For this review, take the finished solid that the model builds, in its own axes (mm). Face numbers are marked on the shaded views. A direction names the side the tool comes from. Coordinates: 2 decimals unless noted, no trailing zeros. Write each loop counter-clockwise with the first axis right and the second up, starting at its lowest first coordinate (ties: lowest second). Pieces come first, ordered by that corner, then holes.
1) Mouldability with a two-part tool opening along Z and no side actions: class the marked faces 1, 2 and 3 as pulls with the +Z half, pulls with the -Z half, needs draft (parallel to the pull), parting line crosses it, or undercut.
2) For the marked faces 4 and 5, list the 3-axis set-ups (+Z, -Z, +X, -X, +Y, -Y) from which the entire face can be reached by the end or side of a thin tool; tool diameter is ignored.
3) We need section A-A on z = 14.35. Write out the cut boundary in (x, y), then the cut area to 3 significant figures.
4) Insertion check: P1, Ø1, axis at x = -11, z = 1, coming from the +Y side; P2, Ø3, axis at x = -13, y = 5.5, coming from the +Z side; P3, Ø5.5, axis at x = 0, y = -5.1, coming from the -Z side. Each pin has a flat end and moves straight along its axis. Give the tip position at first contact, or say it passes through.
5) To check wall thickness, follow line 1 along Y through (x, z) = (0, 32.55); line 2 along Y through (x, z) = (5, -3.4); line 3 along X through (y, z) = (-7.75, 24). State the ranges of each line that lie inside material, in increasing order.
6) We need section B-B on x = 0. Write out the cut boundary in (y, z).
7) We need section C-C on y = 13.25. Write out the cut boundary in (x, z) (3 decimals), then the cut area to 3 significant figures.
8) We need section D-D on x = 7. Write out the cut boundary in (y, z), then the cut area to 3 significant figures.
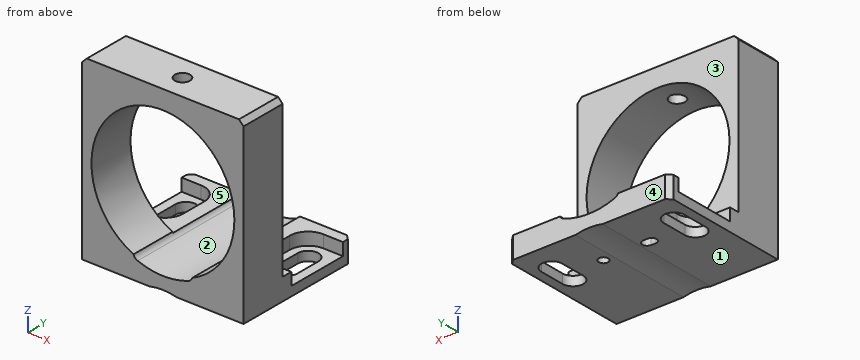
Autodesk Inventor part; units mm, degrees
ref_plane "YZ Plane" through (0, 0, 0) normal (1, 0, 0) x (0, 1, 0)
ref_plane "XZ Plane" through (0, 0, 0) normal (0, 1, 0) x (-1, 0, 0)
ref_plane "XY Plane" through (0, 0, 0) normal (0, 0, 1) x (1, 0, 0)
sketch "Sketch4" plane through (0, 0, 0) normal (0, 0, 1) x (1, 0, 0)
  line L0 (-17.54, 18) -> (17.54, 18)
  line L1 (17.54, 18) -> (17.54, -10.2)
  line L2 (17.54, -10.2) -> (-17.54, -10.2)
  line L3 (-17.54, -10.2) -> (-17.54, 18)
  point P0 (0, 0)
  dimension "d24" = 28.2
  dimension "WIDTH" = 35.08
  dimension "d26" = 17.54
  dimension "d28" = 10.2
extrude "Extrusion3" add sketch "Sketch4" against normal blind 4.7
sketch "Sketch5" plane through (0, 0, 0) normal (0, 0, 1) x (1, 0, 0)
  line L0 (-17.54, -10.2) -> (17.54, -10.2)
  line L1 (17.54, -10.2) -> (17.54, 0)
  line L2 (17.54, 0) -> (-17.54, 0)
  line L3 (-17.54, 0) -> (-17.54, -10.2)
  line L4 (-17.54, 18) -> (-17.54, -10.2)
  line L5 (-17.54, -10.2) -> (17.54, -10.2)
  line L6 (17.54, -10.2) -> (17.54, 18)
  point P0 (0, 0)
  dimension "d31" = 0
  dimension "d32" = 0
  dimension "d33" = 0
  dimension "d34" = 0
extrude "Extrusion4" add sketch "Sketch5" along normal blind 33.93
sketch "Sketch7" plane through (-17.54, -10.2, -4.7) normal (0, -1, 0) x (1, 0, 0)
  circle A0 centre (17.54, 19.05) radius 15.29
  line L0 (35.08, 0) -> (35.08, 38.63)
  line L1 (0, 38.63) -> (35.08, 38.63)
  line L2 (35.08, 0) -> (0, 0)
  line L3 (0, 38.63) -> (0, 0)
  circle A1 centre (17.54, 19.05) radius 15.79
  circle A2 centre (12.6611, 5.6453) radius 1.525
  circle A3 centre (22.4189, 5.6453) radius 1.525
  line L4 (17.54, 19.05) -> (17.54, 6.8001)
  line L5 (12.6611, 5.6453) -> (17.54, 19.05)
  line L6 (22.4189, 5.6453) -> (17.54, 19.05)
  point P0 (22.9405, 4.2123)
  point P1 (21.6565, 4.3246)
  point P2 (13.4235, 4.3246)
  point P3 (12.1395, 4.2123)
  point P4 (23.8519, 5.1236)
  point P5 (11.2281, 5.1236)
  dimension "PILOT_HOLE" = 30.58
  dimension "d201" = 19.05
  dimension "d225" = 17.54
  dimension "d226" = 31.58
  dimension "d227" = 20
  dimension "d228" = 20
  dimension "d229" = 3.05
  dimension "d230" = 3.05
  dimension "d231" = 14.265
  dimension "d232" = 14.265
sketch "Sketch9" plane through (0, 0, -4.7) normal (0, 0, -1) x (-1, 0, 0)
  line L0 (17.54, 18) -> (-17.54, 18)
  line L1 (17.54, 0) -> (-17.54, 0)
  line L2 (0, 5.488) -> (0, 10.988) construction
  line L3 (2.25, 5.488) -> (2.25, 10.988)
  line L4 (-2.25, 10.988) -> (-2.25, 5.488)
  arc A0 (-2.25, 5.488) -> (2.25, 5.488) centre (0, 5.488) ccw
  arc A1 (2.25, 10.988) -> (-2.25, 10.988) centre (0, 10.988) ccw
  line L5 (5.498, 8.238) -> (4.502, 8.238) construction
  line L6 (5.498, 9.288) -> (4.502, 9.288)
  line L7 (4.502, 7.188) -> (5.498, 7.188)
  arc A2 (5.498, 7.188) -> (5.498, 9.288) centre (5.498, 8.238) ccw
  arc A3 (4.502, 9.288) -> (4.502, 7.188) centre (4.502, 8.238) ccw
  point P0 (0, 0)
  point P1 (-5, 8.238)
  point P2 (0, 8.238)
  point P3 (5, 8.238)
  dimension "d183" = 18
  dimension "d185" = 2.25
  dimension "d186" = 5.5
  dimension "d187" = 0
  dimension "d188" = 8.238
  dimension "d189" = 1.05
  dimension "d190" = 0.996
  dimension "d191" = 0
  dimension "d192" = 5
  dimension "d203" = 0
  dimension "d204" = 5
extrude "Extrusion6" cut sketch "Sketch9" against normal blind 2.1 contours A2 L7 A3 L6
extrude "Extrusion7" cut sketch "Sketch7" against normal up to surface (10.2 mm away) contours A0 A3 L6 L5 A2 | A2 A0 | A0 A2 | A3 A0 | A0 A3 | A2 L5 L6 A3 A0 | A0 A3 A1 A2 picked at (17.54, 3.6354)
hole "Hole3" at (5, 8.238, -4.7) direction (0, 0, 1) diameter 2.1 depth 2.1
chamfer "Chamfer10" distance 1 angle 45 4 edges at (17.54, -5.1, 33.93) (-17.54, -5.1, 33.93) (17.54, 18, -2.35) (-17.54, 18, -2.35)
sketch "Sketch13" plane through (-16.54, 18, 0) normal (0, 1, 0) x (1, 0, 0)
  circle A0 centre (16.54, 17.05) radius 12.7
  line L0 (0, 4.7) -> (33.08, 4.7)
  point P0 (16.54, 0)
  dimension "d196" = 0
  dimension "d197" = 25.4
  dimension "d224" = 12.35
extrude "Extrusion11" cut sketch "Sketch13" against normal up to surface (28.2 mm away)
sketch "Sketch14" plane through (0, 0, 33.93) normal (0, 0, 1) x (1, 0, 0)
  line L0 (-17.54, -10.2) -> (17.54, -10.2)
  point P0 (0, 0)
  point P1 (0, -5.1)
  point P2 (-16.54, -10.2)
  point P3 (16.54, -10.2)
  dimension "d212" = 0
  dimension "d213" = 5.1
  dimension "d214" = 10.2
hole "Hole4" at (0, -5.1, 33.93) direction (0, 0, -1) diameter 3.302 end up to surface
sketch "Sketch20" plane through (0, 0, -4.7) normal (0, 0, -1) x (-1, 0, 0)
  line L0 (-17.54, 18) -> (17.54, 18)
  line L1 (-17.54, 0) -> (-17.54, 18)
  line L2 (-13.29, 6.25) -> (-13.29, 11.75) construction
  line L3 (-11.04, 6.25) -> (-11.04, 11.75)
  line L4 (-15.54, 11.75) -> (-15.54, 6.25)
  arc A0 (-15.54, 6.25) -> (-11.04, 6.25) centre (-13.29, 6.25) ccw
  arc A1 (-11.04, 11.75) -> (-15.54, 11.75) centre (-13.29, 11.75) ccw
  line L5 (5.2784, 0) -> (5.2784, 18)
  line L6 (17.54, 18) -> (-17.54, 18)
  line L7 (17.54, -10.2) -> (17.54, 18)
  line L8 (13.29, 6.25) -> (13.29, 11.75) construction
  line L9 (15.54, 6.25) -> (15.54, 11.75)
  line L10 (11.04, 11.75) -> (11.04, 6.25)
  arc A2 (11.04, 6.25) -> (15.54, 6.25) centre (13.29, 6.25) ccw
  arc A3 (15.54, 11.75) -> (11.04, 11.75) centre (13.29, 11.75) ccw
  circle A4 centre (-5, 8.238) radius 1.05
  point P0 (0, 0)
  point P1 (-13.29, 9)
  point P2 (-5.2784, 18)
  point P3 (17.54, 0)
  point P4 (13.29, 9)
  point P5 (16.54, 18)
  dimension "d251" = 18
  dimension "d252" = 9
  dimension "d253" = 12.2616
  dimension "d254" = 4.25
  dimension "d255" = 4.5
  dimension "d256" = 5.5
  dimension "d257" = 18
  dimension "d258" = 12.2616
  dimension "d259" = 9
  dimension "d261" = 4.5
  dimension "d262" = 5.5
  dimension "d293" = 4.25
extrude "Extrusion15" cut sketch "Sketch20" against normal through all contours A0 L4 A1 L3 | A2 L10 A3 L9
sketch "Sketch21" plane through (0, 0, 0) normal (0, 0, 1) x (1, 0, 0)
  line L0 (17.54, 18) -> (-17.54, 18)
  line L1 (17.54, 0) -> (17.54, 18)
  line L2 (17.54, 0) -> (-17.54, 0)
  line L3 (-5.2784, 0) -> (-5.2784, 18)
  line L4 (13.29, 11.75) -> (13.29, 6.25) construction
  line L5 (9.29, 11.75) -> (9.29, 6.25)
  line L6 (17.29, 6.25) -> (17.29, 11.75)
  arc A0 (17.29, 11.75) -> (9.29, 11.75) centre (13.29, 11.75) ccw
  arc A1 (9.29, 6.25) -> (17.29, 6.25) centre (13.29, 6.25) ccw
  line L7 (-13.29, 11.75) -> (-13.29, 6.25) construction
  line L8 (-17.29, 11.75) -> (-17.29, 6.25)
  line L9 (-9.29, 6.25) -> (-9.29, 11.75)
  arc A2 (-9.29, 11.75) -> (-17.29, 11.75) centre (-13.29, 11.75) ccw
  arc A3 (-17.29, 6.25) -> (-9.29, 6.25) centre (-13.29, 6.25) ccw
  line L10 (-17.54, 18) -> (-17.54, 0)
  line L11 (-13.29, 2.25) -> (-17.54, 2.25)
  line L12 (-13.29, 15.75) -> (-17.54, 15.75)
  line L13 (-17.54, -10.2) -> (-17.54, 18)
  line L14 (13.29, 15.75) -> (17.54, 15.75)
  line L15 (13.29, 2.25) -> (17.54, 2.25)
  point P0 (0, 0)
  point P1 (13.29, 9)
  point P2 (5.2784, 18)
  point P3 (-13.29, 9)
  point P4 (-17.54, 15.75)
  point P5 (-16.54, 18)
  dimension "d265" = 9
  dimension "d266" = 4.25
  dimension "d267" = 9
  dimension "d269" = 8
  dimension "d270" = 5.5
  dimension "d271" = 8
  dimension "d272" = 5.5
  dimension "d295" = 4.25
extrude "Extrusion16" cut sketch "Sketch21" against normal blind 2.7 contours L1 L15 A1 L6 A0 L14 | A0 L6 A1 L5 | L12 A2 L8 A3 L11 L10 | A2 L9 A3 L8
sketch "Sketch26" plane through (-17.54, -10.2, -4.7) normal (0, -1, 0) x (1, 0, 0)
  circle A0 centre (17.54, 19.05) radius 15.54
  line L0 (34.4, 0) -> (34.4, 38.38)
  line L1 (0, 38.38) -> (34.4, 38.38)
  line L2 (34.4, 0) -> (0, 0)
  line L3 (0, 0) -> (0, 38.38)
  circle A1 centre (17.54, 19.05) radius 16.04
  circle A2 centre (12.5756, 5.4104) radius 1.525
  circle A3 centre (22.5044, 5.4104) radius 1.525
  line L4 (17.54, 19.05) -> (17.54, 6.8001)
  line L5 (12.5756, 5.4104) -> (17.54, 19.05)
  line L6 (22.5044, 5.4104) -> (17.54, 19.05)
  point P0 (17.54, 4.7)
  point P1 (22.6005, 4.2123)
  point P2 (21.3165, 4.3246)
  point P3 (13.0835, 4.3246)
  point P4 (11.7995, 4.2123)
  point P5 (23.5119, 5.1236)
  point P6 (10.8881, 5.1236)
  point P7 (11.1429, 4.8878)
  point P8 (12.054, 3.9773)
  point P9 (23.026, 3.9773)
  point P10 (23.9371, 4.8878)
  dimension "d314" = 31.08
  dimension "d315" = 19.05
  dimension "d316" = 17.54
  dimension "d317" = 32.08
  dimension "d318" = 20
  dimension "d319" = 20
  dimension "d320" = 3.05
  dimension "d321" = 3.05
  dimension "d322" = 14.515
  dimension "d323" = 14.515
extrude "Extrusion19" cut sketch "Sketch26" against normal through all contours A0 A3 L6 L5 A2 | A2 A0 | A0 A2 | A3 A0 | A0 A3 | A2 L5 L6 A3 A0 | A0 A3 A1 A2 picked at (17.54, 3.3865)
equation "\"TOLERANCE\" = 0.05"
equation "\"BEAM_HEIGHT\" = 19.05"
equation "\"d309\" = 19.05"
equation "\"d311\" = 0.05"
equation "\"d324\" = 19.05"
equation "\"d326\" = 0.05"
properties part number "ADAPTER_SM1L03-new"
Result:
1. face 1: pulls with the -Z half
1. face 2: undercut
1. face 3: needs draft
2. face 4: +Z, -Z, +X, -X, +Y
2. face 5: +Z, +X, -X, +Y
3. outline: (-17.54, -10.2) - (-15.54, -10.2) - (-15.54, 0) - (-17.54, 0) - close; (15.54, -10.2) - (17.54, -10.2) - (17.54, 0) - (15.54, 0) - close
3. area: 40.8 mm2
4. P1: stops at y = 0
4. P2: stops at z = -2.7
4. P3: stops at z = -4.65
5. line 1: y = -10.2 to -6.75, -3.45 to 0
5. line 2: y = -10.2 to 7.19, 9.29 to 18
5. line 3: x = -17.54 to -12.18, 12.18 to 17.54
6. outline: (-10.2, -4.35) - (18, -4.35) - (18, -1.69) - (-10.2, -1.69) - close; (-10.2, 29.89) - (-6.75, 29.89) - (-6.75, 33.93) - (-10.2, 33.93) - close; (-3.45, 29.89) - (0, 29.89) - (0, 33.93) - (-3.45, 33.93) - close
7. outline: (-17.54, -4.7) - (-14.967, -4.7) - (-14.967, -2.7) - (-17.54, -2.7) - close; (-11.613, -4.7) - (-2.961, -4.7) arc R12.7 cw to (2.961, -4.7) - (11.613, -4.7) - (11.613, -2.7) - (9.582, -2.7) - (9.582, 0) - (6.314, 0) arc R1.525 cw to (5.486, -0.723) arc R16.04 cw to (-5.486, -0.723) arc R1.525 cw to (-6.314, 0) - (-9.582, 0) - (-9.582, -2.7) - (-11.613, -2.7) - close; (14.967, -4.7) - (17.54, -4.7) - (17.54, -2.7) - (14.967, -2.7) - close
7. area: 91.3 mm2
8. outline: (-10.2, -4.7) - (18, -4.7) - (18, 0) - (0, 0) - (0, 0.48) - (-10.2, 0.48) - close; (-10.2, 28.22) - (0, 28.22) - (0, 33.93) - (-10.2, 33.93) - close
8. area: 196 mm2
